from build123d import *

# Parameters (mm, degrees)
F0_R     = 2
F1_DEPTH = 0.5


with BuildPart() as f1:
    # F0 (on Front) → F1 (new body, symmetric)
    with BuildSketch(Plane.XZ):
        Polygon((-37.965911, 33.129498), (-37.965911, -30.870502), (-24.465911, -30.870502), (-24.465911, 19.629498), (26.034089, 19.629498), (26.034089, 33.129498), align=None)
        with Locations((-31.215911, -15.870502)):
            Circle(F0_R, mode=Mode.SUBTRACT)
        with Locations((-31.215911, 12.129498)):
            Circle(F0_R, mode=Mode.SUBTRACT)
        with Locations((-16.965911, 26.379498)):
            Circle(F0_R, mode=Mode.SUBTRACT)
        with Locations((11.034089, 26.379498)):
            Circle(F0_R, mode=Mode.SUBTRACT)
    extrude(amount=F1_DEPTH, both=True)


solid = f1.part
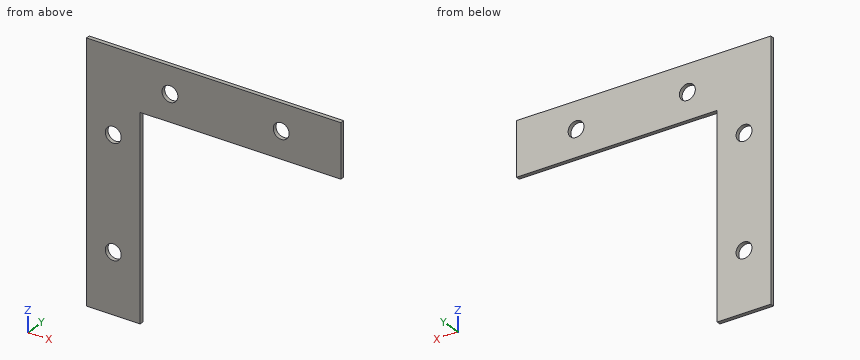
The listing builds one solid part. Answer for the finished solid, in the listing's coordinates (mm). Coordinates: 2 decimals unless noted, no trailing zeros. Loops run counter-clockwise (first coordinate to the right, second up) from the corner with the lowest first, then second, coordinate; pieces in that order, holes last. Notation, with made-up numbers: (87.25, 83) -> (141.25, 83) arc R10 ccw to (141.25, 92) -> close; hole circle Ø11 at (-0.5, -33.5). An arc over 180 degrees is marked (long way). Answer in a Markdown table with one row per item. Add a question column.
1. The part is cut by section D-D, the plane z = -21.5. Write down the section's boundary in (x, y), then the cut area to 3 significant figures.
2. The part is cut by section B-B, the plane y = 0. Write down the section's boundary in (x, z).
3. Consider line 1 (X direction, y = 0, z = 27); line 2 (Z direction, x = -32.5, y = 0.35); line 3 (X direction, y = 0, z = -27). Determine where each line is inside the solid, lowest interval first. Write a range as [from, to].
4. The part is cut by section C-C, the plane x = -10.5. Write down the section's boundary in (y, z), then the cut area to 3 significant figures.
5. The part is cut by section A-A, the plane x = -30. Write down the section's boundary in (y, z), then the cut area to 3 significant figures.
6. A flat-ended cylindrical pin translates along its axis: P1, Ø0.5, axis at y = 0, z = 2, coming from the +X side. Find the tip coordinate at first contact, or state that the pin passes through.
Answer below:
| question | item | result |
|---|---|---|
| 1 | outline | (-37.97, -0.5) -> (-24.47, -0.5) -> (-24.47, 0.5) -> (-37.97, 0.5) -> close |
| 1 | area | 13.5 mm2 |
| 2 | outline | (-37.97, -30.87) -> (-24.47, -30.87) -> (-24.47, 19.63) -> (26.03, 19.63) -> (26.03, 33.13) -> (-37.97, 33.13) -> close; hole circle Ø4 at (-31.22, -15.87); hole circle Ø4 at (-31.22, 12.13); hole circle Ø4 at (-16.97, 26.38); hole circle Ø4 at (11.03, 26.38) |
| 3 | line 1 | [-37.97, -18.87], [-15.06, 9.13], [12.94, 26.03] |
| 3 | line 2 | [-30.87, -17.4], [-14.34, 10.6], [13.66, 33.13] |
| 3 | line 3 | [-37.97, -24.47] |
| 4 | outline | (-0.5, 19.63) -> (0.5, 19.63) -> (0.5, 33.13) -> (-0.5, 33.13) -> close |
| 4 | area | 13.5 mm2 |
| 5 | outline | (-0.5, -30.87) -> (0.5, -30.87) -> (0.5, -17.46) -> (-0.5, -17.46) -> close; (-0.5, -14.28) -> (0.5, -14.28) -> (0.5, 10.54) -> (-0.5, 10.54) -> close; (-0.5, 13.72) -> (0.5, 13.72) -> (0.5, 33.13) -> (-0.5, 33.13) -> close |
| 5 | area | 57.6 mm2 |
| 6 | P1 | x = -24.47 |
